from build123d import *

# Parameters (mm, degrees)
SKETCH_1_W                   = 68
SKETCH_1_H                   = 180
EXTRUDE_1_DEPTH              = 4
HOLE_WIZARD_M2_1_D           = 2.4
HOLE_WIZARD_M2_1_DEPTH       = 7.5
HOLE_WIZARD_M2_1_CSINK_D     = 4.4
HOLE_WIZARD_M2_1_CSINK_ANGLE = 90
HOLE_WIZARD_M2_1_TIP         = 0.721032743
SKETCH_4_R                   = 8.25
CUT_EXTRUDE_1_DEPTH          = 97.291224938
HOLE_WIZARD_M3_1_D           = 3.4
HOLE_WIZARD_M3_1_DEPTH       = 7.5
HOLE_WIZARD_M3_1_CSINK_D     = 6.3
HOLE_WIZARD_M3_1_CSINK_ANGLE = 90
HOLE_WIZARD_M3_1_TIP         = 1.021463052
F_1_0MM_1_D                  = 2.2
SKETCH_17_W                  = 4
SKETCH_17_H                  = 68
EXTRUDE_2_DEPTH              = 3
F_1_0MM_2_D                  = 2.2
F_1_0MM_2_DEPTH              = 6.35
F_1_0MM_2_TIP                = 0.660946681
SKETCH_21_R                  = 5
CUT_EXTRUDE_4_DEPTH          = 100.100958623
F_1_0MM_3_D                  = 2.2
F_1_0MM_3_DEPTH              = 7.25
F_1_0MM_3_TIP                = 0.660946681
F_1_0MM_4_D                  = 2.7


with BuildPart() as part:
    # 草圖1 → 填料-伸長1 (new body)
    with BuildSketch(Plane(origin=(0, 0, 0), x_dir=(0, 0, -1), z_dir=(1, 0, 0))):
        Rectangle(SKETCH_1_W, SKETCH_1_H)
    extrude(amount=EXTRUDE_1_DEPTH)

    # M2 錐坑平頭螺釘的錐孔1
    with Locations(Plane.ZY):
        with Locations((-7.5, 85), (-7.5, 70), (7.5, 85), (7.5, 70)):
            CounterSinkHole(HOLE_WIZARD_M2_1_D / 2, HOLE_WIZARD_M2_1_CSINK_D / 2, depth=HOLE_WIZARD_M2_1_DEPTH, counter_sink_angle=HOLE_WIZARD_M2_1_CSINK_ANGLE)
            with Locations((0, 0, -(HOLE_WIZARD_M2_1_DEPTH + HOLE_WIZARD_M2_1_TIP / 2))):  # 118° drill point
                Cone(0, HOLE_WIZARD_M2_1_D / 2, HOLE_WIZARD_M2_1_TIP, mode=Mode.SUBTRACT)

    # 草圖4 → 除料-伸長1 (cut, through all)
    with BuildSketch(Plane.ZY):
        with Locations((0, 77.5)):
            Circle(SKETCH_4_R)
    extrude(amount=-CUT_EXTRUDE_1_DEPTH, mode=Mode.SUBTRACT)

    # M3 錐坑平頭螺釘的錐孔1
    with Locations(Plane(origin=(4, 0, 0), x_dir=(0, 0, -1), z_dir=(1, 0, 0))):
        with Locations((-25, -30), (0, -30), (25, -30)):
            CounterSinkHole(HOLE_WIZARD_M3_1_D / 2, HOLE_WIZARD_M3_1_CSINK_D / 2, depth=HOLE_WIZARD_M3_1_DEPTH, counter_sink_angle=HOLE_WIZARD_M3_1_CSINK_ANGLE)
            with Locations((0, 0, -(HOLE_WIZARD_M3_1_DEPTH + HOLE_WIZARD_M3_1_TIP / 2))):  # 118° drill point
                Cone(0, HOLE_WIZARD_M3_1_D / 2, HOLE_WIZARD_M3_1_TIP, mode=Mode.SUBTRACT)

    # Ø1.0mm 定位孔1 (through all)
    with Locations(Plane(origin=(4, 0, 0), x_dir=(0, 0, -1), z_dir=(1, 0, 0))):
        with Locations((12, 77.5), (30.5, 77.5)):
            Hole(F_1_0MM_1_D / 2)

    # 草圖17 → 填料-伸長2 (add)
    with BuildSketch(Plane(origin=(0, 90, 0), x_dir=(1, 0, 0), z_dir=(0, 1, 0))):
        with Locations((2, 0)):
            Rectangle(SKETCH_17_W, SKETCH_17_H)
    extrude(amount=EXTRUDE_2_DEPTH)

    # Ø1.0mm 定位孔2
    with Locations(Plane.ZY):
        with Locations((28.7, 88), (28.7, 67), (11.3, 81.6), (11.3, 73.4)):
            Hole(F_1_0MM_2_D / 2, depth=F_1_0MM_2_DEPTH)
            with Locations((0, 0, -(F_1_0MM_2_DEPTH + F_1_0MM_2_TIP / 2))):  # 118° drill point
                Cone(0, F_1_0MM_2_D / 2, F_1_0MM_2_TIP, mode=Mode.SUBTRACT)

    # 草圖21 → 除料-伸長4 (cut, through all)
    with BuildSketch(Plane.ZY):
        with Locations((20, 84.6)):
            Circle(SKETCH_21_R)
        with Locations((20, 70)):
            Circle(SKETCH_21_R)
    extrude(amount=-CUT_EXTRUDE_4_DEPTH, mode=Mode.SUBTRACT)

    # Ø1.0mm 定位孔3
    with Locations(Plane(origin=(0, -90, 0), x_dir=(-1, 0, 0), z_dir=(0, -1, 0))):
        with Locations((-2, 0), (-2, -25), (-2, 25)):
            Hole(F_1_0MM_3_D / 2, depth=F_1_0MM_3_DEPTH)
            with Locations((0, 0, -(F_1_0MM_3_DEPTH + F_1_0MM_3_TIP / 2))):  # 118° drill point
                Cone(0, F_1_0MM_3_D / 2, F_1_0MM_3_TIP, mode=Mode.SUBTRACT)

    # Ø1.0mm 定位孔4 (through all)
    with Locations(Plane(origin=(4, 0, 0), x_dir=(0, 0, -1), z_dir=(1, 0, 0))):
        with Locations((26, -75), (26, 0), (-24, 0), (-24, -75)):
            Hole(F_1_0MM_4_D / 2)


solid = part.part
CAD build for the part. Positions are in the model's coordinates, mm. Give positions to 0.01 mm unless a question says otherwise; leave off trailing zeros. Write each loop counter-clockwise with the first axis right and the second up, starting at its lowest first coordinate (ties: lowest second). Pieces come first, ordered by that corner, then holes. Notation, with made-up numbers: M 89.25,-24.5 L 141.25,-24.5 A10 ccw 141.25,-8.5 Z; hole C 41,-39.5 d11. An arc over 180 degrees is marked long. Put each result on its own line as item: value. Start each with the question number.
(1) Mould opens along Y. For faces 1 (the face through (0, 0, 0)), 2 (the face through (2, 93, 0)), 3 (the face through (1.972, 88.816, 22.688)), 4 (the face through (1.26, -31.66, -0.37)) say: +Y half, -Y half, draft (parallel to the pull), parting line (faces both ways), or undercut.
(2) Band-saw the part on A-A, the plane z = 19. Write the cut outline in (x, y).
(3) Flat gauge pins, fed straight in: pin 1 Ø4.5 at (y, z) = (-30, 25) entering from +X; pin 2 Ø4 at (y, z) = (85, 7.5) entering from -X. Where does each tip first touch, or does it go through?
(4) Probe L1, parallel to Z at x = 2, y = -88.25; L2, parallel to Y at x = 1.35, z = -25; L3, parallel to Z at x = 2.85, y = 73.5. List the from-to ranges inside material, lowest first.
Response values:
1. face 1: draft
1. face 2: +Y half
1. face 3: undercut
1. face 4: undercut
2. outline: M 0,-90 L 4,-90 L 4,65.1 L 0,65.1 Z; M 0,74.9 L 4,74.9 L 4,79.7 L 0,79.7 Z; M 0,89.5 L 4,89.5 L 4,93 L 0,93 Z
3. pin 1: stops at x = 3.1
3. pin 2: stops at x = 0.2
4. L1: z = -34 to -26.1, -23.9 to -1.1, 1.1 to 23.9, 26.1 to 34
4. L2: y = -82.48 to -75.91, -74.09 to -31.7, -28.3 to -0.91, 0.91 to 93
4. L3: z = -34 to -7.22, 7.22 to 10.2, 12.4 to 16.43, 23.57 to 34
